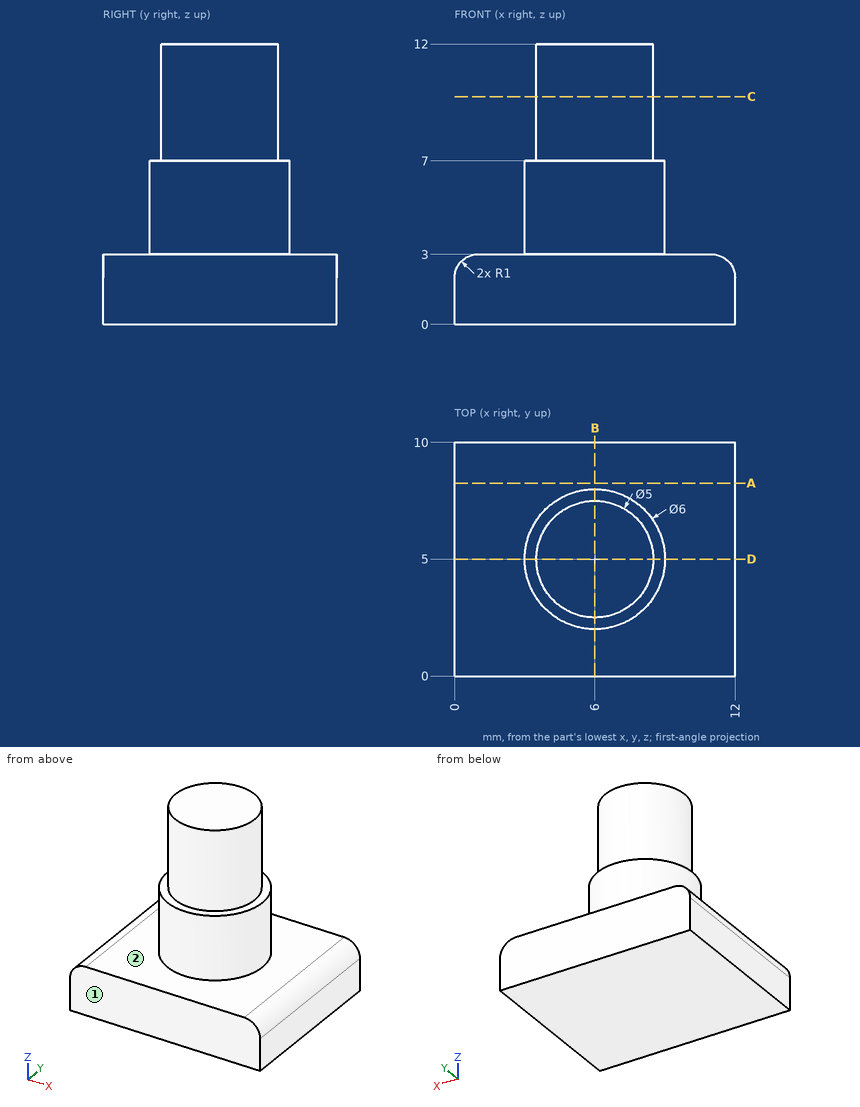
Geometry: see drawing. Coordinates: mm, zero at the bounding-box minimum. A direction names the side the tool comes from. Round coordinates to 2 decimals unless told otherwise and drop trailing zeros. Loops run counter-clockwise (first coordinate to the right, second up) from the corner with the lowest first, then second, coordinate; pieces in that order, holes last. Notation, with made-up numbers: (51.25, -7.5) - (94.25, -7.5) arc R30 ccw to (94.25, 21.5) - close; hole circle Ø3 at (69.5, -4). An arc over 180 degrees is marked (long way). Write item = value, one per line. Start each with the question number.
(1) Section query B-B, the plane x = 6. Output: boundary loops of the cut face in (y, z).
(2) Ray query, line 1 along Z through (x, y) = (8.75, 3.5); line 2 along X through (y, z) = (5, 5.75); line 3 along Z through (x, y) = (7.5, 7.25). Return the intervals inside material, ascending. Write a range as from..to.
(3) Section query C-C, the plane z = 9.75. Output: boundary loops of the cut face in (x, y).
(4) Section query A-A, the plane y = 8.25. Output: boundary loops of the cut face in (x, z), plus the area to 3 significant figures.
(5) Section query D-D, the plane y = 5. Output: boundary loops of the cut face in (x, z).
(6) Set-up query: the marked faces 1 and 2. Return all of +Z, -Z, +X, -X, +Y, -Y with unobstructed straight access to the full face (end or side cutting, diameter ignored); none if empty.
(7) Pin query (flat end, axial travel): pin 1 (3 mm diameter, centred on y = 8.5, z = 7, fed in from -X); pin 2 (1 mm diameter, centred on x = 6, z = 8.5, fed in from +Y); pin 3 (3 mm diameter, centred on x = 9, z = 10, fed in from +Y). Return the tip coordinate at first contact, or that it passes through.
Conclusion:
q1.outline = (0, 0) - (10, 0) - (10, 3) - (8, 3) - (8, 7) - (7.5, 7) - (7.5, 12) - (2.5, 12) - (2.5, 7) - (2, 7) - (2, 3) - (0, 3) - close
q2.line_1 = 0..3
q2.line_2 = 3..9
q2.line_3 = 0..7
q3.outline = circle Ø5 at (6, 5)
q4.outline = (0, 0) - (12, 0) - (12, 2) arc R1 ccw to (11, 3) - (1, 3) arc R1 ccw to (0, 2) - close
q4.area = 35.6 mm2
q5.outline = (0, 0) - (12, 0) - (12, 2) arc R1 ccw to (11, 3) - (9, 3) - (9, 7) - (8.5, 7) - (8.5, 12) - (3.5, 12) - (3.5, 7) - (3, 7) - (3, 3) - (1, 3) arc R1 ccw to (0, 2) - close
q6.face_1 = +Z, -Z, +X, -X, -Y
q6.face_2 = +Z
q7.pin_1 = 3.76
q7.pin_2 = 7.5
q7.pin_3 = 7
